```python
from build123d import *

# Parameters (mm, degrees)
SKETCH_1_R      = 1.05
SKETCH_1_W      = 22
SKETCH_1_H      = 12
EXTRUDE_1_DEPTH = 5.5


with BuildPart() as part:
    # ｽｹｯﾁ1 → ﾎﾞｽ - 押し出し1 (new body)
    with BuildSketch(Plane.XY):
        Polygon((-17, -8), (-7, -8), (-4, -14), (4, -14), (7, -8), (17, -8), (17, 9), (-17, 9), align=None)
        with Locations((-13.7, 0)):
            Circle(SKETCH_1_R, mode=Mode.SUBTRACT)
        with Locations((13.7, 0)):
            Circle(SKETCH_1_R, mode=Mode.SUBTRACT)
        with Locations((0, -10.5)):
            Circle(SKETCH_1_R, mode=Mode.SUBTRACT)
        Rectangle(SKETCH_1_W, SKETCH_1_H, mode=Mode.SUBTRACT)
    extrude(amount=EXTRUDE_1_DEPTH)


solid = part.part
```
Read the model definition and answer for the solid it produces. Units are mm, in the model's axes. A direction names the side the tool comes from. Coordinates: 2 decimals unless noted, no trailing zeros. Loops run counter-clockwise (first coordinate to the right, second up) from the corner with the lowest first, then second, coordinate; pieces in that order, holes last. Notation, with made-up numbers: (35, -34) - (42, -34) arc R17 cw to (42, -18) - close; hole circle Ø8 at (81, 10.5). An arc over 180 degrees is marked (long way). Answer in a Markdown table with one row per item.
1. Which of the six approach directions +Z, -Z, +X, -X, +Y, -Y give full straight-line access (tool end or side, diameter ignored) to faces 1 (the face through (0, 9, 3)), 2 (the face through (12, -8, 3)), 3 (the face through (0, 6, 3))?
Conclusion:
| item | result |
|---|---|
| face 1 | +Z, -Z, +X, -X, +Y |
| face 2 | +Z, -Z, +X, -Y |
| face 3 | +Z, -Z |
2. Find section C-C, the plane x = -10. Write down the section's boundary in (y, z).
Conclusion:
| item | result |
|---|---|
| outline | (-8, 0) - (-6, 0) - (-6, 5.5) - (-8, 5.5) - close; (6, 0) - (9, 0) - (9, 5.5) - (6, 5.5) - close |
3. Find section A-A, the plane x = 0. Write down the section's boundary in (y, z).
Conclusion:
| item | result |
|---|---|
| outline | (-14, 0) - (-11.55, 0) - (-11.55, 5.5) - (-14, 5.5) - close; (-9.45, 0) - (-6, 0) - (-6, 5.5) - (-9.45, 5.5) - close; (6, 0) - (9, 0) - (9, 5.5) - (6, 5.5) - close |
4. Determine the mould class of faces 4 (the face through (0, -6, 3)), 5 (the face through (0, -7, 5.5)), 6 (the face through (-12, -8, 3)) for opening direction Y: +Y half, -Y half, draft (parallel to the pull), parting line (faces both ways), or undercut.
Conclusion:
| item | result |
|---|---|
| face 4 | undercut |
| face 5 | draft |
| face 6 | -Y half |
5. Given pin 1 (1.9 mm diameter, centred on x = -13.7, y = 0, fed in from +Z); pin 2 (2 mm diameter, centred on y = -9.5, z = 3.5, fed in from -X); pin 3 (3 mm diameter, centred on x = 9.5, z = 2.5, fed in from -Y), each flat-ended and moving along its own axis, determine where each tip first touches the part or whether it passes through.
Conclusion:
| item | result |
|---|---|
| pin 1 | passes through |
| pin 2 | stops at x = -6.75 |
| pin 3 | stops at y = -8 |
6. Straight lines are drawn through the part: line 1 (Y direction, x = 0, z = 1.6); line 2 (Y direction, x = 2, z = 3.3); line 3 (X direction, y = -5.5, z = 3.05). For each, find the intervals that lie inside material, in ascending order.
Conclusion:
| item | result |
|---|---|
| line 1 | y = -14 to -11.55, -9.45 to -6, 6 to 9 |
| line 2 | y = -14 to -6, 6 to 9 |
| line 3 | x = -17 to -11, 11 to 17 |
7. Find section B-B, the plane y = 0. Write down the section's boundary in (x, z), then the cut area to 3 significant figures.
Conclusion:
| item | result |
|---|---|
| outline | (-17, 0) - (-14.75, 0) - (-14.75, 5.5) - (-17, 5.5) - close; (-12.65, 0) - (-11, 0) - (-11, 5.5) - (-12.65, 5.5) - close; (11, 0) - (12.65, 0) - (12.65, 5.5) - (11, 5.5) - close; (14.75, 0) - (17, 0) - (17, 5.5) - (14.75, 5.5) - close |
| area | 42.9 mm² |
8. Find section D-D, the plane z = 2.85. Write down the section's boundary in (x, y).
Conclusion:
| item | result |
|---|---|
| outline | (-17, -8) - (-7, -8) - (-4, -14) - (4, -14) - (7, -8) - (17, -8) - (17, 9) - (-17, 9) - close; hole circle Ø2.1 at (-13.7, 0); hole (-11, -6) - (11, -6) - (11, 6) - (-11, 6) - close; hole circle Ø2.1 at (0, -10.5); hole circle Ø2.1 at (13.7, 0) |
